Part model, mm, in its own coordinate system. A direction names the side the tool comes from. Round coordinates to 2 decimals unless told otherwise and drop trailing zeros. Order: outer loops, then holes, each group sorted by start corner. A loop starts at its lowest first (then second) coordinate and runs counter-clockwise, first axis right, second up. Notation, with made-up numbers: (61, -35.5) - (65, -35.5) arc R24 ccw to (65, -7.5) - close; hole circle Ø6 at (71.25, -8). An arc over 180 degrees is marked (long way). Return JSON: item names as keys, results as strings. Group by question number.
Item 1: Two-plate mould, pull along Y, no slides. Class faces 1 (the face through (92, 29, 0)), 2 (the face through (28.503, 74.128, 12.522)), 3 (the face through (26.4, 50, 13)), 4 (the face through (75, 0, 13)): released by +Y, released by -Y, zero draft, split by the parting line, or undercut.
Item 2: Saw through at B-B on x = 92.5. List the corners of the cut face in (y, z), and give its area (3 significant figures).
Item 3: Saw through at C-C on z = 20.75. List the corners of the cut face in (x, y), and give its area (3 significant figures).
Item 4: Tool access for faces 5 (the face through (75, 101.6, 13)), 6 (the face through (62.15, 22.434, 12.522)): list every direction of +Z, -Z, +X, -X, +Y, -Y with a clear straight run to the whole face (end or side of a thin tool).
Item 5: Saw through at A-A on y = 64. List the corners of the cut face in (x, z), and give its area (3 significant figures).
Item 6: Probe probe 1 along Y at (x, z) = (62.5, 7.25); probe 2 along X at (y, z) = (72, 6.25); probe 3 along Y at (x, z) = (47.5, 22.75). List the from-to ranges inside material, lowest first.
```python
from build123d import *

# Parameters (mm, degrees)
F0_W     = 152.4
F0_H     = 101.6
F1_DEPTH = 25.4
F3_DEPTH = 25.4
F4_R     = 7.62


with BuildPart() as f1:
    # F0 (on Top) → F1 (new body)
    with BuildSketch(Plane.XY):
        with Locations((76.2, 50.8)):
            Rectangle(F0_W, F0_H)
    extrude(amount=F1_DEPTH)

    # F2 (on face) → F3 (cut)
    with BuildSketch(Plane.XY.offset(25.4)):
        Polygon((138.869882, 83.813608), (26.399821, 75.979866), (26.399821, 22.262821), (62.211186, 22.262821), (138.869882, 57.514634), align=None)
    extrude(amount=-F3_DEPTH, mode=Mode.SUBTRACT)

    # F4
    f4_edges = [f1.edges().sort_by_distance(p)[0] for p in [
        (26.399821, 75.979866, 12.7),
        (26.399821, 22.262821, 12.7),
        (62.211186, 22.262821, 12.7),
        (138.869882, 57.514634, 12.7),
        (138.869882, 83.813608, 12.7),
    ]]
    fillet(f4_edges, radius=F4_R)


solid = f1.part
```
Filled in:
{
 "1": {"face 1": "zero draft", "face 2": "undercut", "face 3": "undercut", "face 4": "released by -Y"},
 "2": {"outline": "(0, 0) - (36.19, 0) - (36.19, 25.4) - (0, 25.4) - close; (80.58, 0) - (101.6, 0) - (101.6, 25.4) - (80.58, 25.4) - close", "area": "1,450 mm^2"},
 "3": {"outline": "(0, 0) - (152.4, 0) - (152.4, 101.6) - (0, 101.6) - close; hole (26.4, 29.88) arc R7.62 ccw to (34.02, 22.26) - (60.54, 22.26) arc R7.62 ccw to (63.73, 22.96) - (134.43, 55.47) arc R7.62 ccw to (138.87, 62.4) - (138.87, 75.64) arc R7.62 ccw to (130.72, 83.25) - (33.49, 76.47) arc R7.62 ccw to (26.4, 68.87) - close", "area": "10,400 mm^2"},
 "4": {"face 5": "+Z, -Z, +X, -X, +Y", "face 6": "+Z, -Z"},
 "5": {"outline": "(0, 0) - (26.4, 0) - (26.4, 25.4) - (0, 25.4) - close; (138.87, 0) - (152.4, 0) - (152.4, 25.4) - (138.87, 25.4) - close", "area": "1,010 mm^2"},
 "6": {"probe 1": "y = 0 to 22.52, 78.49 to 101.6", "probe 2": "x = 0 to 27.07, 138.87 to 152.4", "probe 3": "y = 0 to 22.26, 77.45 to 101.6"}
}
